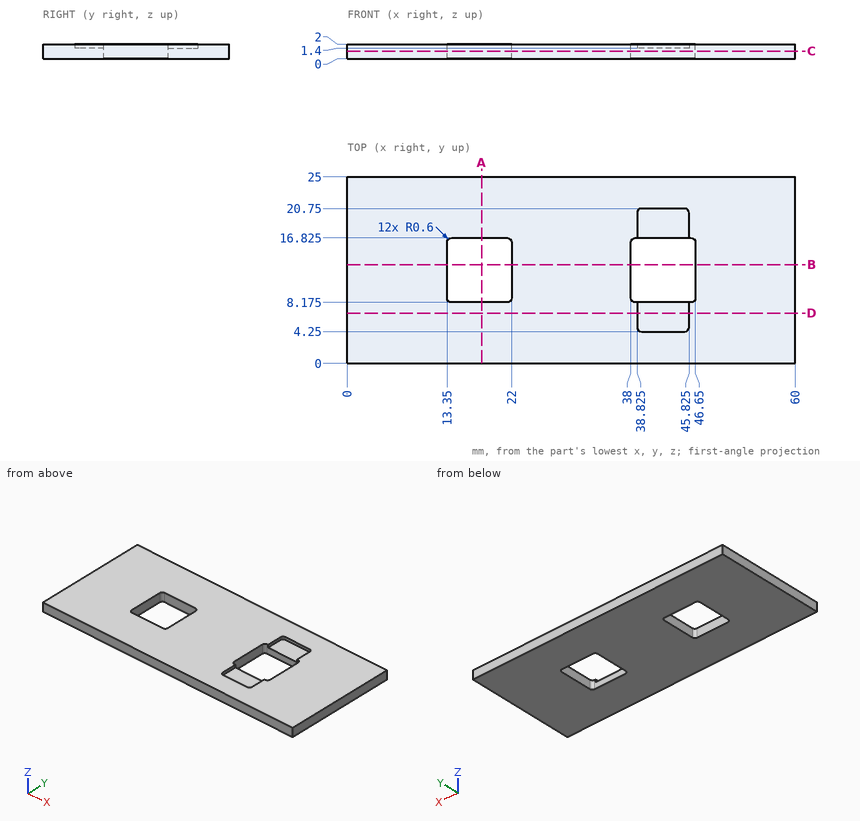
Answer from the drawing. Dimensions are ordinates in mm from the lowest x, y and z of the part. Give positions to 0.01 mm unless a question says otherwise; leave off trailing zeros. Loops run counter-clockwise (first coordinate to the right, second up) from the corner with the lowest first, then second, coordinate; pieces in that order, holes last. Notation, with made-up numbers: (-32.5, 86.5) - (17.5, 86.5) arc R18 cw to (17.5, 121.5) - close; hole circle Ø7 at (30, -27.5). An arc over 180 degrees is marked (long way). Answer as CSV lines item,"result". Start each with the question number.
Item 1: A cutting plane is placed at C-C on z = 1.05. Determine the outline of the cut face in (x, y) (3 decimals), then the cut area to 3 significant figures.
Item 2: Each of these flat-tipped pins is pushed along its axis until it touches: pin 1 (4 mm diameter, centred on x = 41, y = 10.5, fed in from -Z); pin 2 (1.2 mm diameter, centred on x = 41, y = 18.5, fed in from +Z). Where does it stop, or does it pass through?
Item 3: Find the intervals of material crossed by line 1 (X direction, y = 13, z = 1.15); line 2 (Y direction, x = 19.5, z = 0.75) (3 decimals); line 3 (Z direction, x = 39.5, y = 18), in increasing order. Write a range as from..to.
Item 4: A cutting plane is placed at A-A on x = 18. Determine the outline of the cut face in (y, z) (3 decimals), then the cut area to 3 significant figures.
Item 5: A cutting plane is placed at D-D on y = 6.75. Determine the outline of the cut face in (x, z) (3 decimals), then the cut area to 3 significant figures.
Item 6: A cutting plane is placed at B-B on y = 13.25. Determine the outline of the cut face in (x, z).
Found:
1,outline,"(0, 0) - (60, 0) - (60, 25) - (0, 25) - close; hole (13.35, 8.775) arc R0.6 ccw to (13.95, 8.175) - (21.4, 8.175) arc R0.6 ccw to (22, 8.775) - (22, 16.225) arc R0.6 ccw to (21.4, 16.825) - (13.95, 16.825) arc R0.6 ccw to (13.35, 16.225) - close; hole (38, 8.775) arc R0.6 ccw to (38.6, 8.175) - (46.05, 8.175) arc R0.6 ccw to (46.65, 8.775) - (46.65, 16.225) arc R0.6 ccw to (46.05, 16.825) - (38.6, 16.825) arc R0.6 ccw to (38, 16.225) - close"
1,area,"1,350 mm^2"
2,pin 1,"passes through"
2,pin 2,"stops at z = 1.4"
3,line 1,"x = 0..13.35, 22..38, 46.65..60"
3,line 2,"y = 0..8.175, 16.825..25"
3,line 3,"z = 0..1.4"
4,outline,"(0, 0) - (8.175, 0) - (8.175, 2) - (0, 2) - close; (16.825, 0) - (25, 0) - (25, 2) - (16.825, 2) - close"
4,area,"32.7 mm^2"
5,outline,"(0, 0) - (60, 0) - (60, 2) - (45.825, 2) - (45.825, 1.4) - (38.825, 1.4) - (38.825, 2) - (0, 2) - close"
5,area,"116 mm^2"
6,outline,"(0, 0) - (13.35, 0) - (13.35, 2) - (0, 2) - close; (22, 0) - (38, 0) - (38, 2) - (22, 2) - close; (46.65, 0) - (60, 0) - (60, 2) - (46.65, 2) - close"
